Verification items for this drawing (mm, ordinates from the low corner). A direction names the side the tool comes from. Give positions to 0.01 mm unless a question says otherwise; leave off trailing zeros. Loops run counter-clockwise (first coordinate to the right, second up) from the corner with the lowest first, then second, coordinate; pieces in that order, holes last. Notation, with made-up numbers: M 4.5,30 L 19.5,30 A31 ccw 19.5,60 Z; hole C 32.25,-12 d3. An arc over 180 degrees is marked long. Use one line per item in the form item = value.
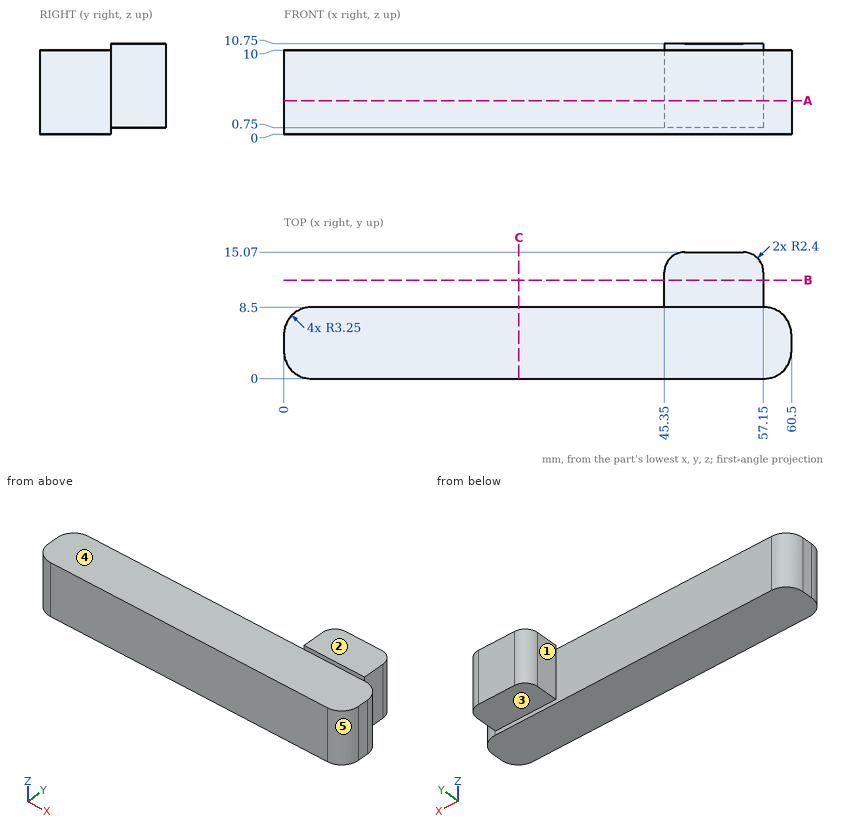
1) Set-up check for the marked faces 1, 2, 3, 4 and 5: record each of +Z, -Z, +X, -X, +Y, -Y from which the full face is reachable in a straight line by a thin tool's end or side.
Evaluation:
face_1 = +Z, -Z, -X, +Y
face_2 = +Z, +X, -X, +Y, -Y
face_3 = -Z, +X, -X, +Y
face_4 = +Z, +X, -X, -Y
face_5 = +Z, -Z, +X, -Y
2) Depth check by flat-ended pin: pin 1 Ø1 at (y, z) = (6, 2.5) entering from +X; pin 2 Ø3 at (x, z) = (28.5, 3) entering from +Y; pin 3 Ø1 at (y, z) = (8, 4.5) entering from +X. Enter the tip coordinate at first touch or a pass-through.
Evaluation:
pin_1 = 60.49
pin_2 = 8.5
pin_3 = 59.6
3) Section check A-A (z = 4). Record the cut outline in (x, y), then the cut area to 3 significant figures.
Evaluation:
outline = M 0,3.25 A3.25 ccw 3.25,0 L 57.25,0 A3.25 ccw 60.5,3.25 L 60.5,5.25 A3.25 ccw 57.25,8.5 L 57.15,8.5 L 57.15,12.67 A2.4 ccw 54.75,15.07 L 47.75,15.07 A2.4 ccw 45.35,12.67 L 45.35,8.5 L 3.25,8.5 A3.25 ccw 0,5.25 Z
area = 580 mm^2
4) Scan lines: line 1 (Z direction, x = 46, y = 12.75); line 2 (Y direction, x = 37.5, z = 2.75); line 3 (Z direction, x = 26, y = 8.25). Record each from-to range of solid material in increasing order.
Evaluation:
line_1 = 0.75 to 10.75
line_2 = 0 to 8.5
line_3 = 0 to 10
5) Section check C-C (x = 28). Record the cut outline in (y, z).
Evaluation:
outline = M 0,0 L 8.5,0 L 8.5,10 L 0,10 Z
6) Section check B-B (y = 11.75). Record the cut outline in (x, z), then the cut area to 3 significant figures.
Evaluation:
outline = M 45.35,0.75 L 57.15,0.75 L 57.15,10.75 L 45.35,10.75 Z
area = 118 mm^2
